from build123d import *

# Parameters (mm, degrees)
SKETCH1_R           = 12.75
BOSS_EXTRUDE1_DEPTH = 6.35
FILLET1_R           = 1
FILLET2_R           = 1


with BuildPart() as part:
    # Sketch1 → Boss-Extrude1 (new body)
    with BuildSketch(Plane(origin=(0, 0, 0), x_dir=(1, 0, 0), z_dir=(0, 1, 0))):
        with Locations(Location((0, 0, 0), (0, 0, 270))):
            Circle(SKETCH1_R)
        with BuildLine():
            Line((1.411048864, 1.6), (-1.411048864, 1.6))
            ThreePointArc((-1.411048864, 1.6), (-2.617971935, 2.994195507), (-2.768208587, 1.156296337))
            ThreePointArc((-2.768208587, 1.156296337), (0, -3), (2.768208587, 1.156296337))
            ThreePointArc((2.768208587, 1.156296337), (2.617971935, 2.994195507), (1.411048864, 1.6))
        make_face(mode=Mode.SUBTRACT)
    extrude(amount=BOSS_EXTRUDE1_DEPTH)

    # Fillet1
    fillet1_edges = [part.edges().sort_by_distance(p)[0] for p in [
        (2.768208587, 3.175, -1.156296337),
        (1.411048864, 3.175, -1.6),
        (-1.411048864, 3.175, -1.6),
        (-2.768208587, 3.175, -1.156296337),
    ]]
    fillet(fillet1_edges, radius=FILLET1_R)

    # Fillet2
    fillet2_edges = [part.edges().sort_by_distance(p)[0] for p in [
        (0, 0, -12.75),
        (0, 6.35, -12.75),
    ]]
    fillet(fillet2_edges, radius=FILLET2_R)


solid = part.part
Part model, mm, in its own coordinate system. Give positions to 0.01 mm unless a question says otherwise; leave off trailing zeros. Write each loop counter-clockwise with the first axis right and the second up, starting at its lowest first coordinate (ties: lowest second). Pieces come first, ordered by that corner, then holes.
1) Pin check, flat tip, straight feed: pin 1 (2 mm diameter, centred on x = 5, y = 5, fed in from -Z). Stop position of the tip, or through.
Resolved:
pin 1: stops at z = -12.11
2) Cut at A-A on x = 0. Write the cut outline in (y, z).
Resolved:
outline: (0, -11.75) arc R1 ccw to (1, -12.75) - (5.35, -12.75) arc R1 ccw to (6.35, -11.75) - (6.35, -1.6) - (0, -1.6) - close; (0, 3) - (6.35, 3) - (6.35, 11.75) arc R1 ccw to (5.35, 12.75) - (1, 12.75) arc R1 ccw to (0, 11.75) - close
3) Probe L1, parallel to X at y = 3.75, z = 0; L2, parallel to X at y = 0.5, z = -1.75; L3, parallel to X at y = 2, z = -1.5. List the from-to ranges inside material, lowest first.
Resolved:
L1: x = -12.75 to -3, 3 to 12.75
L2: x = -12.49 to -3.26, -0.91 to 0.91, 3.26 to 12.49
L3: x = -12.66 to -3.15, 3.15 to 12.66
4) Cut at B-B on z = 0. Write the cut outline in (x, y).
Resolved:
outline: (-12.75, 1) arc R1 ccw to (-11.75, 0) - (-3, 0) - (-3, 6.35) - (-11.75, 6.35) arc R1 ccw to (-12.75, 5.35) - close; (3, 0) - (11.75, 0) arc R1 ccw to (12.75, 1) - (12.75, 5.35) arc R1 ccw to (11.75, 6.35) - (3, 6.35) - close
